The model under review builds one solid part; all positions refer to its coordinate system, in mm. A direction names the side the tool comes from. Coordinates: 2 decimals unless noted, no trailing zeros. Order: outer loops, then holes, each group sorted by start corner. A loop starts at its lowest first (then second) coordinate and runs counter-clockwise, first axis right, second up. Notation, with made-up numbers: (50.25, -29.5) -> (106.25, -29.5) arc R22 cw to (106.25, -12.5) -> close; hole circle Ø8 at (45, -3.5). An arc over 180 degrees is marked (long way). Put each result on its own line as item: value.
from build123d import *

# Parameters (mm, degrees)
SKETCH_1_W          = 41.58
SKETCH_1_H          = 4.8
SKETCH_1_R          = 1.15
EXTRUDE_1_DEPTH     = 3
SKETCH_2_R          = 2.05
CUT_EXTRUDE_1_DEPTH = 1.2
SKETCH_3_W          = 3
SKETCH_3_H          = 4.8
EXTRUDE_2_DEPTH     = 5


with BuildPart() as part:
    # 草图1 → 凸台-拉伸1 (new body)
    with BuildSketch(Plane(origin=(0, 0, 0), x_dir=(0, 0, -1), z_dir=(1, 0, 0))):
        with Locations((20.79, 2.4)):
            Rectangle(SKETCH_1_W, SKETCH_1_H)
        with Locations((14.79, 2.4)):
            Circle(SKETCH_1_R, mode=Mode.SUBTRACT)
        with Locations((5.79, 2.4)):
            Circle(SKETCH_1_R, mode=Mode.SUBTRACT)
        with Locations(Location((26.79, 2.4, 0), (0, 0, 180))):
            Circle(SKETCH_1_R, mode=Mode.SUBTRACT)
        with Locations(Location((35.79, 2.4, 0), (0, 0, 180))):
            Circle(SKETCH_1_R, mode=Mode.SUBTRACT)
    extrude(amount=EXTRUDE_1_DEPTH)

    # 草图2 → 切除-拉伸1 (cut)
    with BuildSketch(Plane(origin=(3, 0, 0), x_dir=(0, 0, -1), z_dir=(1, 0, 0))):
        with Locations((5.79, 2.4)):
            Circle(SKETCH_2_R)
        with Locations((14.79, 2.4)):
            Circle(SKETCH_2_R)
        with Locations((26.79, 2.4)):
            Circle(SKETCH_2_R)
        with Locations((35.79, 2.4)):
            Circle(SKETCH_2_R)
    extrude(amount=-CUT_EXTRUDE_1_DEPTH, mode=Mode.SUBTRACT)

    # 草图3 → 凸台-拉伸2 (add)
    with BuildSketch(Plane.XY):
        with Locations((1.5, 2.4)):
            Rectangle(SKETCH_3_W, SKETCH_3_H)
    extrude(amount=EXTRUDE_2_DEPTH)


solid = part.part
Item 1: Consider section C-C on x = 2.2. Write out the cut boundary in (y, z), and give its area (3 significant figures).
Answers below:
outline: (0, -41.58) -> (4.8, -41.58) -> (4.8, 5) -> (0, 5) -> close; hole circle Ø4.1 at (2.4, -35.79); hole circle Ø4.1 at (2.4, -26.79); hole circle Ø4.1 at (2.4, -14.79); hole circle Ø4.1 at (2.4, -5.79)
area: 171 mm^2
Item 2: Consider section B-B on x = 0.55. Write out the cut boundary in (y, z).
Answers below:
outline: (0, -41.58) -> (4.8, -41.58) -> (4.8, 5) -> (0, 5) -> close; hole circle Ø2.3 at (2.4, -35.79); hole circle Ø2.3 at (2.4, -26.79); hole circle Ø2.3 at (2.4, -14.79); hole circle Ø2.3 at (2.4, -5.79)
Item 3: Consider section A-A on z = -26.79. Write out the cut boundary in (x, y), and give its area (3 significant figures).
Answers below:
outline: (0, 0) -> (3, 0) -> (3, 0.35) -> (1.8, 0.35) -> (1.8, 1.25) -> (0, 1.25) -> close; (0, 3.55) -> (1.8, 3.55) -> (1.8, 4.45) -> (3, 4.45) -> (3, 4.8) -> (0, 4.8) -> close
area: 5.34 mm^2
Item 4: Mouldability with a two-part tool opening along Z and no side actions: class faces 3 (the flat face through (1.8, 2.4, -28.1)), 4 (the flat face through (3, 2, -19)), 5 (the flat face through (1, 2, -41.58)) as +Z half, -Z half, draft (parallel to the pull), parting line (faces both ways), or undercut.
Answers below:
face 3: undercut
face 4: draft
face 5: -Z half
Item 5: For line 1 (Z direction, x = 1.4, y = 2.4); line 2 (Z direction, x = 2, y = 2.7); line 3 (Y direction, x = 2.65, z = -5.79), list the stretches that pass through material, from the lowest coordinate up. Write a range as from..to.
Answers below:
line 1: -41.58..-36.94, -34.64..-27.94, -25.64..-15.94, -13.64..-6.94, -4.64..5
line 2: -41.58..-37.82, -33.76..-28.82, -24.76..-16.82, -12.76..-7.82, -3.76..5
line 3: 0..0.35, 4.45..4.8
Item 6: For faces 1 (the flat face through (1, 0, -19)), 2 (the cylindrical face through (2.41, 2.49, -24.74)), list the 3-axis set-ups (+Z, -Z, +X, -X, +Y, -Y) from which the entire face can be reached by the end or side of a thin tool; tool diameter is ignored.
Answers below:
face 1: +Z, -Z, +X, -X, -Y
face 2: +X
Item 7: For pin 1 Ø2 at (y, z) = (2.4, -35.79) entering from +X; pin 2 Ø2 at (y, z) = (3, -36.5) entering from +X, all flat-tipped, find the tip position at first contact; note any pin that passes through.
Answers below:
pin 1: through
pin 2: x = 1.8
Item 8: Consider section D-D on y = 2.9. Count the separate pieces of the cut face and the enclosed holes in it, and give its area (3 significant figures).
Answers below:
separate pieces: 5
enclosed holes: 0
area: 106 mm^2
